```python
from build123d import *

# Parameters (mm, degrees)
F1_DEPTH = 127
F3_DEPTH = 88.901
F5_DEPTH = 63.501
F6_R     = 9.92251
F7_DEPTH = 88.901
F8_R     = 10.3251
F9_DEPTH = 25.4


with BuildPart() as f1:
    # F0 (on Right) → F1 (new body)
    with BuildSketch(Plane.YZ):
        with BuildLine():
            Line((-76.2, 0), (-12.7, 0))
            ThreePointArc((-12.7, 0), (-3.719744, 3.719744), (0, 12.7))
            Line((0, 12.7), (0, 63.5))
            Line((0, 63.5), (-7.9375, 63.5))
            Line((-7.9375, 63.5), (-7.9375, 12.7))
            ThreePointArc((-7.9375, 12.7), (-9.332404, 9.332404), (-12.7, 7.9375))
            Line((-12.7, 7.9375), (-76.2, 7.9375))
            ThreePointArc((-76.2, 7.9375), (-79.567596, 9.332404), (-80.9625, 12.7))
            Line((-80.9625, 12.7), (-80.9625, 63.5))
            Line((-80.9625, 63.5), (-88.9, 63.5))
            Line((-88.9, 63.5), (-88.9, 12.7))
            ThreePointArc((-88.9, 12.7), (-85.180256, 3.719744), (-76.2, 0))
        make_face()
    extrude(amount=F1_DEPTH)

    # F2 (on face) → F3 (cut, through all)
    with BuildSketch(Plane.XZ.offset(88.9)):
        with BuildLine():
            Line((0, 63.5), (0, 34.925))
            ThreePointArc((0, 34.925), (8.369424, 55.130576), (28.575, 63.5))
            Line((28.575, 63.5), (0, 63.5))
        make_face()
        with BuildLine():
            ThreePointArc((28.575, 63.5), (48.780576, 55.130576), (57.15, 34.925))
            Line((57.15, 34.925), (57.15, 63.5))
            Line((57.15, 63.5), (28.575, 63.5))
        make_face()
    extrude(amount=-F3_DEPTH, mode=Mode.SUBTRACT)

    # F4 (on face) → F5 (cut, through all)
    with BuildSketch(Plane.XY.offset(63.5)):
        with BuildLine():
            Line((127, 0), (57.15, 0))
            Line((57.15, 0), (57.15, -15.945885))
            ThreePointArc((57.15, -15.945885), (59.01373, -20.439868), (63.510907, -22.295876))
            Line((63.510907, -22.295876), (104.775, -22.225))
            ThreePointArc((104.775, -22.225), (120.490448, -28.734552), (127, -44.45))
            Line((127, -44.45), (127, 0))
        make_face()
        with BuildLine():
            Line((127, -88.9), (127, -44.45))
            ThreePointArc((127, -44.45), (120.490448, -60.165448), (104.775, -66.675))
            Line((104.775, -66.675), (63.510907, -66.604124))
            ThreePointArc((63.510907, -66.604124), (59.01373, -68.460132), (57.15, -72.954115))
            Line((57.15, -72.954115), (57.15, -88.9))
            Line((57.15, -88.9), (127, -88.9))
        make_face()
    extrude(amount=-F5_DEPTH, mode=Mode.SUBTRACT)

    # F6 (on face) → F7 (cut, through all)
    with BuildSketch(Plane.XZ.offset(88.9)):
        with Locations((28.575, 44.45)):
            Circle(F6_R)
    extrude(amount=-F7_DEPTH, mode=Mode.SUBTRACT)

    # F8 (on face) → F9 (cut)
    with BuildSketch(Plane.XY.offset(7.9375)):
        with Locations((73.025, -44.45)):
            Circle(F8_R)
        with Locations((111.125, -44.45)):
            Circle(F8_R)
    extrude(amount=-F9_DEPTH, mode=Mode.SUBTRACT)


solid = f1.part
```
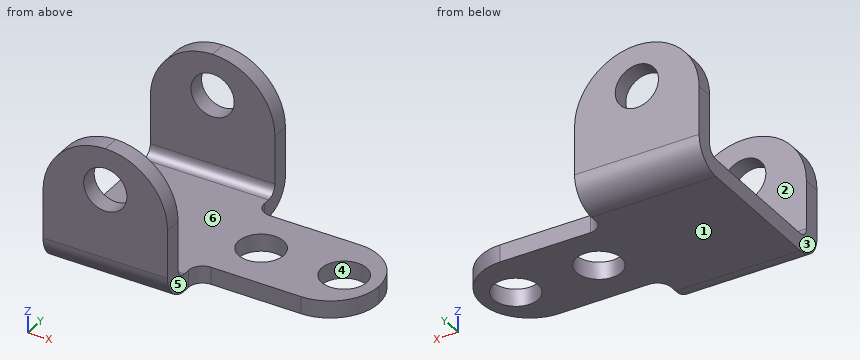
Check sheet for the modelled part. Datum: model origin and axes. Units: mm. Face numbers are marked on the shaded views. A direction names the side the tool comes from. Coordinates: 2 decimals unless noted, no trailing zeros. Loops run counter-clockwise (first coordinate to the right, second up) from the corner with the lowest first, then second, coordinate; pieces in that order, holes last.
1) Sectioned sample at C-C (x = 20.5). Record the boundary of the cut face in (y, z) (1 decimal), and give its area (3 significant figures).
2) Gauge pin test, flat ends, axial feed: pin 1 (17.5 mm diameter, centred on y = -80, z = 21.5, fed in from +X); pin 2 (12 mm diameter, centred on x = 21, z = 47, fed in from +Y); pin 3 (23.5 mm diameter, centred on x = 73.025, y = -44.45, fed in from +Z). Record the tip position at first contact, or that the pin passes through.
3) Material ranges on probe 1 along Y at (x, z) = (40.5, 43.5); probe 2 along Z at (x, y) = (6, -39.5); probe 3 along Z at (x, y) = (6, -80.5), recorded low to high.
4) Sectioned sample at A-A (x = 78.5). Record the boundary of the cut face in (y, z), and give its area (3 significant figures).
5) Release check for a two-part mould opening along X. For the marked faces 3, 4, 5 and 6 record: released by +X, released by -X, zero draft, split by the parting line, or undercut.
6) Access from +Z, -Z, +X, -X, +Y, -Y to the whole of each face (thin tool, end or side, straight path). Record for the marked faces 1 and 2.
7) Sectioned sample at B-B (z = 59). Record the boundary of the cut face in (x, y), and give its area (3 significant figures).
8) Sectioned sample at D-D (y = -42). Record the boundary of the cut face in (x, z), and give its area (3 significant figures).
Check sheet entries:
1. outline: (-88.9, 12.7) arc R12.7 ccw to (-76.2, 0) - (-12.7, 0) arc R12.7 ccw to (0, 12.7) - (0, 38.7) - (-7.9, 38.7) - (-7.9, 12.7) arc R4.8 cw to (-12.7, 7.9) - (-76.2, 7.9) arc R4.8 cw to (-81, 12.7) - (-81, 38.7) - (-88.9, 38.7) - close; (-88.9, 50.2) - (-81, 50.2) - (-81, 62.3) - (-88.9, 62.3) - close; (-7.9, 50.2) - (0, 50.2) - (0, 62.3) - (-7.9, 62.3) - close
1. area: 1,330 mm2
2. pin 1: stops at x = 57.15
2. pin 2: stops at y = 0
2. pin 3: stops at z = 7.94
3. probe 1: y = -88.9 to -80.96, -7.94 to 0
3. probe 2: z = 0 to 7.94
3. probe 3: z = 0.75 to 10.65
4. outline: (-66.63, 0) - (-53.2, 0) - (-53.2, 7.94) - (-66.63, 7.94) - close; (-35.7, 0) - (-22.27, 0) - (-22.27, 7.94) - (-35.7, 7.94) - close
4. area: 213 mm2
5. face 3: released by -X
5. face 4: undercut
5. face 5: released by +X
5. face 6: zero draft
6. face 1: -Z, +X, -X, +Y, -Y
6. face 2: +Z, +X, -X
7. outline: (13.18, -88.9) - (43.97, -88.9) - (43.97, -80.96) - (13.18, -80.96) - close; (13.18, -7.94) - (43.97, -7.94) - (43.97, 0) - (13.18, 0) - close
7. area: 489 mm2
8. outline: (0, 0) - (62.99, 0) - (62.99, 7.94) - (0, 7.94) - close; (83.06, 0) - (101.09, 0) - (101.09, 7.94) - (83.06, 7.94) - close; (121.16, 0) - (126.86, 0) - (126.86, 7.94) - (121.16, 7.94) - close
8. area: 689 mm2
